Check sheet for the modelled part. Datum: model origin and axes. Units: mm. Round coordinates to 2 decimals unless told otherwise and drop trailing zeros. Write each loop counter-clockwise with the first axis right and the second up, starting at its lowest first coordinate (ties: lowest second). Pieces come first, ordered by that corner, then holes. Notation, with made-up numbers: M -8.75,-39 L 41.25,-39 A21 ccw 41.25,-15 Z; hole C -7.75,-16.5 d6. An arc over 180 degrees is marked long. Put each result on its own line as item: value.
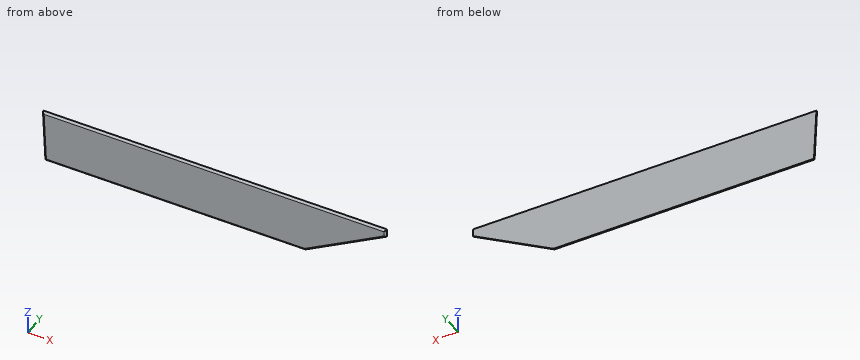
```python
from build123d import *

# Parameters (mm, degrees)
F1_DEPTH = 6.35
F2_R     = 5


with BuildPart() as f1:
    # F0 (on Front) → F1 (new body)
    with BuildSketch(Plane.XZ):
        Polygon((372.662067, 966.672301), (-550.337933, 966.672301), (-543.763254, 827.127099), (156.236746, 827.127099), (372.662067, 946.672301), align=None)
    extrude(amount=F1_DEPTH)

    # F2
    f2_edges = [f1.edges().sort_by_distance(p)[0] for p in [
        (264.449407, -6.35, 886.8997),
        (372.662067, -6.35, 956.672301),
        (-88.837933, -6.35, 966.672301),
        (-547.050593, -6.35, 896.8997),
        (-193.763254, -6.35, 827.127099),
    ]]
    fillet(f2_edges, radius=F2_R)


solid = f1.part
```
1. Scan lines: probe 1 along Z at (x, y) = (-253, -1.75); probe 2 along X at (y, z) = (-5, 851.5); probe 3 along X at (y, z) = (-0.75, 955). Record each from-to range of solid material in increasing order.
Computed values:
probe 1: z = 827.14 to 966.66
probe 2: x = -543.33 to 197.09
probe 3: x = -549.79 to 372.66
2. Cross-section at A-A (y = -3.25). Enter the section's corners in (x, z), then the cut area to 3 significant figures.
Computed values:
outline: M -549.94,966.3 L -543.41,827.5 L 156.14,827.5 L 372.29,946.89 L 372.29,966.3 Z
area: 115,000 mm2
3. Depth check by flat-ended pin: pin 1 Ø1.5 at (y, z) = (-1, 950.5) entering from -X. Enter the tip coordinate at first touch or a pass-through.
Computed values:
pin 1: stops at x = -549.61
